```python
from build123d import *

# Parameters (mm, degrees)
BOSS_EXTRUDE1_DEPTH = 7.25
BOSS_EXTRUDE2_DEPTH = 1.1
FILLET1_R           = 0.5
SKETCH4_W           = 90
SKETCH4_H           = 15.8
BOSS_EXTRUDE3_DEPTH = 7.25
FILLET3_R           = 0.5
BOSS_EXTRUDE4_DEPTH = 7.25


with BuildPart() as part:
    # Sketch1 → Boss-Extrude1 (new body)
    with BuildSketch(Plane(origin=(0, 0, 0), x_dir=(1, 0, 0), z_dir=(0, 1, 0))):
        with BuildLine():
            Line((0, 0), (18.25, 0))
            ThreePointArc((18.25, 0), (18.603553391, 0.146446609), (18.75, 0.5))
            Line((18.75, 0.5), (18.75, 5))
            ThreePointArc((18.75, 5), (18.603553391, 5.353553391), (18.25, 5.5))
            Line((18.25, 5.5), (3.85, 5.5))
            ThreePointArc((3.85, 5.5), (3.496446609, 5.646446609), (3.35, 6))
            Line((3.35, 6), (3.35, 7.2))
            ThreePointArc((3.35, 7.2), (3.496446609, 7.553553391), (3.85, 7.7))
            Line((3.85, 7.7), (18.25, 7.7))
            ThreePointArc((18.25, 7.7), (18.603553391, 7.846446609), (18.75, 8.2))
            Line((18.75, 8.2), (18.75, 12.7))
            ThreePointArc((18.75, 12.7), (18.603553391, 13.053553391), (18.25, 13.2))
            Line((18.25, 13.2), (0, 13.2))
            Line((0, 13.2), (0, 0))
        make_face()
    extrude(amount=BOSS_EXTRUDE1_DEPTH)

    # Sketch2 → Boss-Extrude2 (add)
    with BuildSketch(Plane(origin=(0, 7.25, 0), x_dir=(1, 0, 0), z_dir=(0, 1, 0))):
        with BuildLine():
            Line((1.25, 3.55), (16.85, 3.55))
            ThreePointArc((16.85, 3.55), (17.65, 2.75), (16.85, 1.95))
            Line((16.85, 1.95), (1.25, 1.95))
            ThreePointArc((1.25, 1.95), (0.45, 2.75), (1.25, 3.55))
        make_face()
        with BuildLine():
            Line((1.25, 9.65), (16.85, 9.65))
            ThreePointArc((16.85, 9.65), (17.65, 10.45), (16.85, 11.25))
            Line((16.85, 11.25), (1.25, 11.25))
            ThreePointArc((1.25, 11.25), (0.45, 10.45), (1.25, 9.65))
        make_face()
    extrude(amount=BOSS_EXTRUDE2_DEPTH)

    # Fillet1
    fillet1_edges = [part.edges().sort_by_distance(p)[0] for p in [
        (18.603553391, 7.25, -0.146446609),
        (18.75, 7.25, -2.75),
        (18.603553391, 7.25, -5.353553391),
        (11.05, 7.25, -5.5),
        (3.496446609, 7.25, -5.646446609),
        (3.35, 7.25, -6.6),
        (3.496446609, 7.25, -7.553553391),
        (11.05, 7.25, -7.7),
        (18.603553391, 7.25, -7.846446609),
        (0.45, 8.35, -2.75),
        (9.05, 8.35, -1.95),
        (17.65, 8.35, -2.75),
        (9.05, 8.35, -3.55),
        (18.75, 7.25, -10.45),
        (18.603553391, 7.25, -13.053553391),
        (9.125, 7.25, -13.2),
        (0.45, 8.35, -10.45),
        (9.05, 8.35, -9.65),
        (17.65, 8.35, -10.45),
        (9.05, 8.35, -11.25),
        (9.125, 7.25, 0),
    ]]
    fillet(fillet1_edges, radius=FILLET1_R)

    # Sketch4 → Boss-Extrude3 (add)
    with BuildSketch(Plane(origin=(0, 0, 0), x_dir=(1, 0, 0), z_dir=(0, 1, 0))):
        with Locations((-45, 6.6)):
            Rectangle(SKETCH4_W, SKETCH4_H)
    extrude(amount=BOSS_EXTRUDE3_DEPTH)

    # Fillet3
    # the kernel refuses this fillet: 0.5 mm, written as the material it adds along each edge
    with BuildSketch(Plane(origin=(0, 0, 0), x_dir=(0, 0, 1), z_dir=(0, 1, 0))) as fillet3_piece_1:
        with BuildLine():
            CenterArc((FILLET3_R, FILLET3_R), FILLET3_R, 180, 90)
            Line((0, FILLET3_R), (0, 0))
            Line((0, 0), (FILLET3_R, 0))
        make_face()
    extrude(amount=6.75)
    with BuildSketch(Plane(origin=(0, 0, -13.2), x_dir=(0, 0, -1), z_dir=(0, 1, 0))) as fillet3_piece_2:
        with BuildLine():
            CenterArc((FILLET3_R, -FILLET3_R), FILLET3_R, 90, 90)
            Line((0, -FILLET3_R), (0, 0))
            Line((0, 0), (FILLET3_R, 0))
        make_face()
    extrude(amount=6.75)
    with BuildSketch(Plane(origin=(0, 6.75, -12.7), x_dir=(0, -0.8017442392976486, 0.5976672776328271), z_dir=(0, -0.5976672776328271, -0.8017442392976486))) as fillet3_piece_3_section:
        with BuildLine():
            CenterArc((0.5 + FILLET3_R, -FILLET3_R), FILLET3_R, 90, 90)
            Line((0.5, -FILLET3_R), (0.5, 0))
            Line((0.5, 0), (0.5 + FILLET3_R, 0))
        make_face()
    fillet3_piece_3 = revolve(axis=Axis((0, 6.75, -12.7), (-1, 0, 0)), revolution_arc=233.296989237, mode=Mode.PRIVATE)
    fillet3_piece_3 = split(fillet3_piece_3, bisect_by=Plane(origin=(0.15581414, 7.25, -13.074969472), z_dir=(0, -1, 0)), keep=Keep.TOP, mode=Mode.PRIVATE)
    add(fillet3_piece_3)
    with BuildSketch(Plane(origin=(0, 6.75, -0.5), x_dir=(0, -0.801744239297648, -0.5976672776328278), z_dir=(0, -0.5976672776328278, 0.801744239297648))) as fillet3_piece_4_section:
        with BuildLine():
            CenterArc((0.5 + FILLET3_R, FILLET3_R), FILLET3_R, 180, 90)
            Line((0.5, FILLET3_R), (0.5, 0))
            Line((0.5, 0), (0.5 + FILLET3_R, 0))
        make_face()
    fillet3_piece_4 = revolve(axis=Axis((0, 6.75, -0.5), (1, 0, 0)), revolution_arc=233.296989237, mode=Mode.PRIVATE)
    fillet3_piece_4 = split(fillet3_piece_4, bisect_by=Plane(origin=(0.155814151, 7.25, -0.125030527), z_dir=(0, -1, 0)), keep=Keep.TOP, mode=Mode.PRIVATE)
    add(fillet3_piece_4)
    # the kernel refuses this fillet: 0.5 mm, written as the material it takes off along each edge
    with BuildSketch(Plane(origin=(0, -1.25, 1.3), x_dir=(0, 0, -1), z_dir=(0, 1, 0))) as fillet3_2_piece_1:
        with BuildLine():
            CenterArc((FILLET3_R, FILLET3_R), FILLET3_R, 180, 90)
            Line((0, FILLET3_R), (0, 0))
            Line((0, 0), (FILLET3_R, 0))
        make_face()
    extrude(amount=9.75, mode=Mode.SUBTRACT)
    with BuildSketch(Plane(origin=(0, -1.25, -14.5), x_dir=(0, 0, 1), z_dir=(0, 1, 0))) as fillet3_2_piece_2:
        with BuildLine():
            CenterArc((FILLET3_R, -FILLET3_R), FILLET3_R, 90, 90)
            Line((0, -FILLET3_R), (0, 0))
            Line((0, 0), (FILLET3_R, 0))
        make_face()
    extrude(amount=9.75, mode=Mode.SUBTRACT)
    with BuildSketch(Plane(origin=(-91.25, 7.25, 1.3), x_dir=(0, 0, -1), z_dir=(1, 0, 0)), Plane(origin=(1.25, 7.25, -14.5), x_dir=(0, 0, 1), z_dir=(-1, 0, 0))) as fillet3_2_piece_3:
        with BuildLine():
            CenterArc((FILLET3_R, -FILLET3_R), FILLET3_R, 90, 90)
            Line((0, -FILLET3_R), (0, 0))
            Line((0, 0), (FILLET3_R, 0))
        make_face()
    extrude(amount=92.5, mode=Mode.SUBTRACT)

    # Sketch5 → Boss-Extrude4 (add)
    with BuildSketch(Plane(origin=(0, 7.25, 0), x_dir=(1, 0, 0), z_dir=(0, 1, 0))):
        with BuildLine():
            Line((-90, 14.5), (-91.694558873, 15.893887447))
            ThreePointArc((-91.694558873, 15.893887447), (-101.255273326, 22.85289034), (-111.570616913, 28.634643431))
            Line((-111.570616913, 28.634643431), (-127.809202797, 36.513023717))
            ThreePointArc((-127.809202797, 36.513023717), (-133.229461338, 35.472077659), (-133.770408027, 29.979341726))
            ThreePointArc((-133.770408027, 29.979341726), (-133.726831866, 27.027184623), (-136.276459546, 25.538383383))
            Line((-136.276459546, 25.538383383), (-149.666955308, 25.538383383))
            ThreePointArc((-149.666955308, 25.538383383), (-153.346325023, 22.325436822), (-150.658389652, 18.246737208))
            ThreePointArc((-150.658389652, 18.246737208), (-149.277221775, 16.150939464), (-151.167827967, 14.5))
            ThreePointArc((-151.167827967, 14.5), (-154.994699417, 10.67312855), (-151.167827967, 6.8462571))
            ThreePointArc((-151.167827967, 6.8462571), (-149.535956381, 5.487012057), (-150.577779387, 3.636294146))
            ThreePointArc((-150.577779387, 3.636294146), (-153.292773274, -1.415823247), (-148.677747615, -4.821204301))
            Line((-148.677747615, -4.821204301), (-129.766646687, -3.335569849))
            ThreePointArc((-129.766646687, -3.335569849), (-125.233182835, -6.296372519), (-126.944947273, -11.433347257))
            Line((-126.944947273, -11.433347257), (-130.743308987, -13.988655394))
            ThreePointArc((-130.743308987, -13.988655394), (-132.049672504, -20.665923892), (-125.372404006, -21.97228741))
            Line((-125.372404006, -21.97228741), (-109.093123035, -11.020571314))
            ThreePointArc((-109.093123035, -11.020571314), (-99.841658682, -5.580656509), (-90, -1.3))
            Line((-90, -1.3), (-90, 14.5))
        make_face()
    extrude(amount=-BOSS_EXTRUDE4_DEPTH)


solid = part.part
```
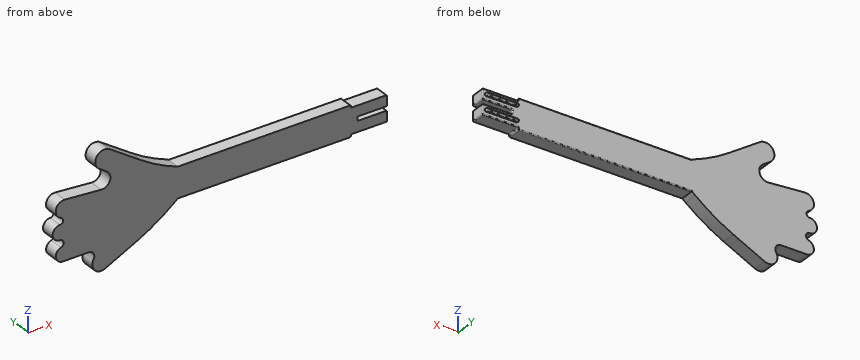
Geometry: final body of the model. Coordinates: model frame, mm. Coordinates: 2 decimals unless noted, no trailing zeros. Order: outer loops, then holes, each group sorted by start corner. A loop starts at its lowest first (then second) coordinate and runs counter-clockwise, first axis right, second up.
Item 1: Contact query for flat-ended pins moving along their axis: P1, Ø0.6, axis at y = 7, z = -14.5, coming from the +X side; P2, Ø5, axis at y = 1, z = -5, coming from the -X side; P3, Ø2, axis at x = -141.5, y = 5, coming from the -Z side; P4, Ø1, axis at x = -120, z = -30, coming from the -Y side. Output: stop coordinate, or through.
Answer:
P1: stops at x = -0.04
P2: stops at x = -153.31
P3: stops at z = -25.54
P4: stops at y = 0
Item 2: Section query C-C (x = -139). Output: boundary loops of the cut face in (y, z), then the cut area to 3 significant figures.
Answer:
outline: (0, -25.54) - (7.25, -25.54) - (7.25, 4.06) - (0, 4.06) - close
area: 215 mm2
Item 3: Material intervals for line 1 along Z through (x, y) = (8, 2); line 2 along Z through (x, y) = (-63, 6); line 3 along Y through (x, z) = (-123, 9), sorted ascending.
Answer:
line 1: z = -13.2 to -7.7, -5.5 to 0
line 2: z = -14.5 to 1.3
line 3: y = 0 to 7.25
Item 4: Section query B-B (z = -21). Output: boundary loops of the cut face in (x, y), then the cut area to 3 significant figures.
Answer:
outline: (-153.29, 0) - (-98.47, 0) - (-98.47, 7.25) - (-153.29, 7.25) - close
area: 397 mm2
Item 5: Section query A-A (x = -78.5). Output: boundary loops of the cut face in (y, z), then the cut area to 3 significant figures.
Answer:
outline: (0, -14.5) - (6.75, -14.5) arc R0.5 ccw to (7.25, -14) - (7.25, 0.8) arc R0.5 ccw to (6.75, 1.3) - (0, 1.3) - close
area: 114 mm2
